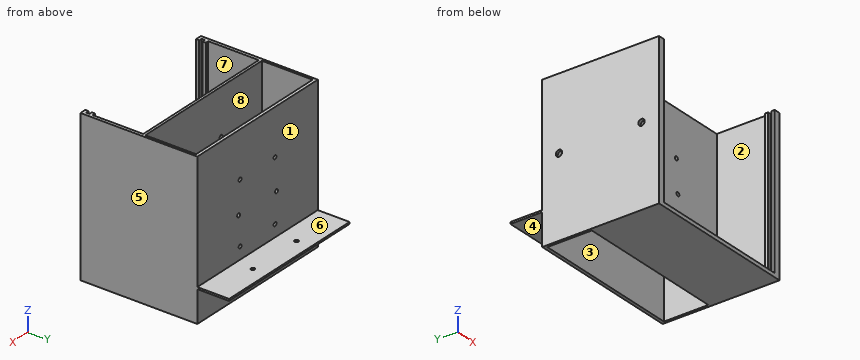
```python
from build123d import *

# Parameters (mm, degrees)
SKETCH_2_W          = 124
SKETCH_2_H          = 120
EXTRUDE_1_DEPTH     = 2
SKETCH_3_W          = 2
SKETCH_3_H          = 120
EXTRUDE_2_DEPTH     = 40
SKETCH_4_W          = 120
SKETCH_4_H          = 2
EXTRUDE_3_DEPTH     = 5
SKETCH_6_W          = 124
SKETCH_6_H          = 120
EXTRUDE_4_DEPTH     = 2.5
SKETCH_9_W          = 124
SKETCH_9_H          = 1.5
EXTRUDE_5_DEPTH     = 25
SKETCH_10_R         = 1.5
CUT_EXTRUDE_2_DEPTH = 1.5
SKETCH_11_R         = 1.5
CUT_EXTRUDE_3_DEPTH = 51
SKETCH_12_W         = 2.5
SKETCH_12_H         = 120
EXTRUDE_6_DEPTH     = 47.5
SKETCH_14_W         = 2.5
SKETCH_14_H         = 2.5
EXTRUDE_8_DEPTH     = 120
SKETCH_15_W         = 119
SKETCH_15_H         = 3
EXTRUDE_9_DEPTH     = 47.5
SKETCH_16_R         = 2.5
CUT_EXTRUDE_4_DEPTH = 10
SKETCH_18_W         = 2.5
SKETCH_18_H         = 2.5
EXTRUDE_10_DEPTH    = 120


with BuildPart() as part:
    # 草图2 → 凸台-拉伸1 (new body)
    with BuildSketch(Plane(origin=(0, 0, 0), x_dir=(1, 0, 0), z_dir=(0, 1, 0))):
        Rectangle(SKETCH_2_W, SKETCH_2_H)
    extrude(amount=EXTRUDE_1_DEPTH)

    # 草图3 → 凸台-拉伸2 (add)
    with BuildSketch(Plane(origin=(0, 2, 0), x_dir=(1, 0, 0), z_dir=(0, 1, 0))):
        with Locations((-61, 0)):
            Rectangle(SKETCH_3_W, SKETCH_3_H)
        with Locations((61, 0)):
            Rectangle(SKETCH_3_W, SKETCH_3_H)
    extrude(amount=EXTRUDE_2_DEPTH)

    # 草图4 → 凸台-拉伸3 (add)
    with BuildSketch(Plane(origin=(0, 2, 0), x_dir=(1, 0, 0), z_dir=(0, 1, 0))):
        with Locations((0, 59)):
            Rectangle(SKETCH_4_W, SKETCH_4_H)
    extrude(amount=EXTRUDE_3_DEPTH)

    # 草图6 → 凸台-拉伸4 (add)
    with BuildSketch(Plane(origin=(0, 42, 0), x_dir=(1, 0, 0), z_dir=(0, 1, 0))):
        Rectangle(SKETCH_6_W, SKETCH_6_H)
    extrude(amount=EXTRUDE_4_DEPTH)

    # 草图9 → 凸台-拉伸5 (add)
    with BuildSketch(Plane(origin=(0, 44.5, 0), x_dir=(1, 0, 0), z_dir=(0, 1, 0))):
        with Locations((0, 34.25)):
            Rectangle(SKETCH_9_W, SKETCH_9_H)
    extrude(amount=EXTRUDE_5_DEPTH)

    # 草图10 → 切除-拉伸2 (cut)
    with BuildSketch(Plane(origin=(0, 0, -35), x_dir=(-1, 0, 0), z_dir=(0, 0, -1))):
        with Locations((-22.5, 58)):
            Circle(SKETCH_10_R)
        with Locations((22.5, 58)):
            Circle(SKETCH_10_R)
    extrude(amount=-CUT_EXTRUDE_2_DEPTH, mode=Mode.SUBTRACT)

    # 草图11 → 切除-拉伸3 (cut)
    with BuildSketch(Plane(origin=(0, 44.5, 0), x_dir=(1, 0, 0), z_dir=(0, 1, 0))):
        with Locations(Location((-19.5, 1, 0), (0, 0, 270))):
            Circle(SKETCH_11_R)
        with Locations(Location((-18, 24, 0), (0, 0, 270))):
            Circle(SKETCH_11_R)
        with Locations(Location((-18, -24, 0), (0, 0, 270))):
            Circle(SKETCH_11_R)
        with Locations(Location((18, -24, 0), (0, 0, 270))):
            Circle(SKETCH_11_R)
        with Locations(Location((19.5, 1, 0), (0, 0, 270))):
            Circle(SKETCH_11_R)
        with Locations(Location((18, 24, 0), (0, 0, 270))):
            Circle(SKETCH_11_R)
    extrude(amount=-CUT_EXTRUDE_3_DEPTH, mode=Mode.SUBTRACT)

    # 草图12 → 凸台-拉伸6 (add)
    with BuildSketch(Plane.XZ):
        with Locations((-60.75, 0)):
            Rectangle(SKETCH_12_W, SKETCH_12_H)
        with Locations((60.75, 0)):
            Rectangle(SKETCH_12_W, SKETCH_12_H)
    extrude(amount=EXTRUDE_6_DEPTH)

    # 草图14 → 凸台-拉伸8 (add)
    with BuildSketch(Plane(origin=(0, 0, -60), x_dir=(-1, 0, 0), z_dir=(0, 0, -1))):
        with Locations((-58.25, -46.25)):
            Rectangle(SKETCH_14_W, SKETCH_14_H)
        with Locations((58.25, -46.25)):
            Rectangle(SKETCH_14_W, SKETCH_14_H)
    extrude(amount=-EXTRUDE_8_DEPTH)

    # 草图15 → 凸台-拉伸9 (add)
    with BuildSketch(Plane.XZ):
        with Locations((0, -58.5)):
            Rectangle(SKETCH_15_W, SKETCH_15_H)
    extrude(amount=EXTRUDE_9_DEPTH)

    # 草图16 → 切除-拉伸4 (cut)
    with BuildSketch(Plane.ZY.offset(62)):
        with Locations((2.778789214, 31.36631919)):
            Circle(SKETCH_16_R)
        with Locations((2.778789214, -33.63368081)):
            Circle(SKETCH_16_R)
    extrude(amount=-CUT_EXTRUDE_4_DEPTH, mode=Mode.SUBTRACT)

    # 草图18 → 凸台-拉伸10 (add)
    with BuildSketch(Plane.XY.offset(60)):
        with Locations((-58.25, -41.1)):
            Rectangle(SKETCH_18_W, SKETCH_18_H)
        with Locations((58.25, -41.1)):
            Rectangle(SKETCH_18_W, SKETCH_18_H)
    extrude(amount=-EXTRUDE_10_DEPTH)


solid = part.part
```
CAD build for the part. Positions are in the model's coordinates, mm. Face numbers are marked on the shaded views. A direction names the side the tool comes from. Coordinates: 2 decimals unless noted, no trailing zeros. Order: outer loops, then holes, each group sorted by start corner. A loop starts at its lowest first (then second) coordinate and runs counter-clockwise, first axis right, second up. Notation, with made-up numbers: (50, 4.5) -> (59, 4.5) arc R11 cw to (59, 10.5) -> close; hole circle Ø8 at (8, 67.5). An arc over 180 degrees is marked (long way). Use one line per item in the form item = value. Start each with the question number.
1) Band-saw the part on A-A on x = 7. Give the cut face in (y, z).
2) Drop flat-ended pins along their axis: pin 1 (24 mm diameter, centred on x = 6.5, y = -17.5, fed in from +Z); pin 2 (2 mm diameter, centred on x = 6.5, z = 22.5, fed in from +Y); pin 3 (7.5 mm diameter, centred on x = -6.5, y = 53.5, fed in from +Z); pin 4 (2.5 mm diameter, centred on x = 18, z = 24, fed in from +Y). Give the stop position or say it passes through.
3) Band-saw the part on B-B on z = -45. Give the cut face in (x, y).
4) Band-saw the part on C-C on y = 9.5. Give the cut face in (x, z).
5) Band-saw the part on D-D on y = -2.5. Give the cut face in (x, z).
6) Pull direction X, two halves, no side cores. Call the marked faces 5, 6, 7 and 8: +X half, -X half, draft (parallel to the pull), parting line (faces both ways), or undercut.
7) Tool access for the marked faces 1, 2, 3 and 4: list every direction of +Z, -Z, +X, -X, +Y, -Y with a clear straight run to the whole face (end or side of a thin tool).
8) Drill centre lines: L1, parallel to X at y = 43, z = 24; L2, parallel to X at y = 43, z = -1; L3, parallel to Y at x = 22.5, z = -33.75. Where is each one in solid material? Low to high. Write a range as [from, to].
Entries:
q1.outline = (-47.5, -60) -> (7, -60) -> (7, -58) -> (2, -58) -> (2, 60) -> (0, 60) -> (0, -57) -> (-47.5, -57) -> close; (42, -60) -> (44.5, -60) -> (44.5, -35) -> (69.5, -35) -> (69.5, -33.5) -> (44.5, -33.5) -> (44.5, 60) -> (42, 60) -> close
q2.pin_1 = -57
q2.pin_2 = 44.5
q2.pin_3 = -33.5
q2.pin_4 = through
q3.outline = (-62, -47.5) -> (-57, -47.5) -> (-57, -45) -> (-59.5, -45) -> (-59.5, -42.35) -> (-57, -42.35) -> (-57, -39.85) -> (-59.5, -39.85) -> (-59.5, 0) -> (59.5, 0) -> (59.5, -39.85) -> (57, -39.85) -> (57, -42.35) -> (59.5, -42.35) -> (59.5, -45) -> (57, -45) -> (57, -47.5) -> (62, -47.5) -> (62, 44.5) -> (-62, 44.5) -> close; hole (-60, 2) -> (60, 2) -> (60, 42) -> (-60, 42) -> close
q4.outline = (-62, -60) -> (-60, -60) -> (-60, 60) -> (-62, 60) -> close; (60, -60) -> (62, -60) -> (62, 60) -> (60, 60) -> close
q5.outline = (-62, -60) -> (62, -60) -> (62, 60) -> (59.5, 60) -> (59.5, -57) -> (-59.5, -57) -> (-59.5, 60) -> (-62, 60) -> close
q6.face_5 = +X half
q6.face_6 = draft
q6.face_7 = undercut
q6.face_8 = undercut
q7.face_1 = +Z, +X, -X, +Y
q7.face_2 = +Z
q7.face_3 = +Z, -Z
q7.face_4 = -Z, +X, -X, +Y
q8.L1 = [-62, -19.5], [-16.5, 16.5], [19.5, 62]
q8.L2 = [-62, -21], [-18, 18], [21, 62]
q8.L3 = [0, 2], [42, 56.5], [59.5, 69.5]
